from build123d import *

# Parameters (mm, degrees)
F0_R           = 0.875
F1_DEPTH       = 12.6
F2_DEPTH       = 2
F4_D           = 2
F4_DEPTH       = 38
F4_CBORE_D     = 3.5
F4_CBORE_DEPTH = 3
F4_TIP         = 0.600860619


# Not quite as in the source:
# - a feature names something its author has since deleted; it is built from what else it names


with BuildPart() as f1:
    # F0 (on Front) → F1 (new body)
    with BuildSketch(Plane.XZ):
        with BuildLine():
            Line((1, 0), (6.25, 0))
            Line((6.25, 0), (4.5, 17.15))
            Line((4.5, 17.15), (0, 17.15))
            Line((0, 17.15), (-4.5, 17.15))
            Line((-4.5, 17.15), (-6.25, 0))
            Line((-6.25, 0), (-1, 0))
            Line((-1, 0), (-1, 3))
            Line((-1, 3), (-3.25, 3))
            ThreePointArc((-3.25, 3), (-4.75, 4.5), (-3.25, 6))
            Line((-3.25, 6), (0, 6))
            Line((0, 6), (3.25, 6))
            ThreePointArc((3.25, 6), (4.75, 4.5), (3.25, 3))
            Line((3.25, 3), (1, 3))
            Line((1, 3), (1, 0))
        make_face()
        with Locations((-2.675, 9.625)):
            Circle(F0_R, mode=Mode.SUBTRACT)
        with Locations((2.675, 9.625)):
            Circle(F0_R, mode=Mode.SUBTRACT)
        with BuildLine():
            Line((-2.5, 16.4487531745), (0, 16.4487531745))
            Line((0, 16.4487531745), (2.5, 16.4487531745))
            ThreePointArc((2.5, 16.4487531745), (3.5, 15.4487531745), (2.5, 14.4487531745))
            Line((2.5, 14.4487531745), (0, 14.4487531745))
            Line((0, 14.4487531745), (-2.5, 14.4487531745))
            ThreePointArc((-2.5, 14.4487531745), (-3.5, 15.4487531745), (-2.5, 16.4487531745))
        make_face(mode=Mode.SUBTRACT)
        with BuildLine():
            Line((2.5, 16.4487531745), (0, 16.4487531745))
            Line((0, 16.4487531745), (-2.5, 16.4487531745))
            ThreePointArc((-2.5, 16.4487531745), (-3.5, 15.4487531745), (-2.5, 14.4487531745))
            Line((-2.5, 14.4487531745), (0, 14.4487531745))
            Line((0, 14.4487531745), (2.5, 14.4487531745))
            ThreePointArc((2.5, 14.4487531745), (3.5, 15.4487531745), (2.5, 16.4487531745))
        make_face()
        with Locations((-2.675, 9.625)):
            Circle(F0_R)
        with Locations((2.675, 9.625)):
            Circle(F0_R)
        with BuildLine():
            Line((1, 3.65), (1, 3))
            Line((1, 3), (3.25, 3))
            ThreePointArc((3.25, 3), (4.75, 4.5), (3.25, 6))
            Line((3.25, 6), (0, 6))
            Line((0, 6), (-3.25, 6))
            ThreePointArc((-3.25, 6), (-4.75, 4.5), (-3.25, 3))
            Line((-3.25, 3), (-1, 3))
            Line((-1, 3), (-1, 3.65))
            Line((-1, 3.65), (0, 3.65))
            Line((0, 3.65), (1, 3.65))
        make_face()
    extrude(amount=-F1_DEPTH)

    # F0 (on Front) → F2 (cut)
    with BuildSketch(Plane.XZ):
        with BuildLine():
            Line((1, 3.65), (1, 3))
            Line((1, 3), (3.25, 3))
            ThreePointArc((3.25, 3), (4.75, 4.5), (3.25, 6))
            Line((3.25, 6), (0, 6))
            Line((0, 6), (-3.25, 6))
            ThreePointArc((-3.25, 6), (-4.75, 4.5), (-3.25, 3))
            Line((-3.25, 3), (-1, 3))
            Line((-1, 3), (-1, 3.65))
            Line((-1, 3.65), (0, 3.65))
            Line((0, 3.65), (1, 3.65))
        make_face()
        with BuildLine():
            Line((2.5, 16.4487531745), (0, 16.4487531745))
            Line((0, 16.4487531745), (-2.5, 16.4487531745))
            ThreePointArc((-2.5, 16.4487531745), (-3.5, 15.4487531745), (-2.5, 14.4487531745))
            Line((-2.5, 14.4487531745), (0, 14.4487531745))
            Line((0, 14.4487531745), (2.5, 14.4487531745))
            ThreePointArc((2.5, 14.4487531745), (3.5, 15.4487531745), (2.5, 16.4487531745))
        make_face()
        with Locations((2.675, 9.625)):
            Circle(F0_R)
        with Locations((-2.675, 9.625)):
            Circle(F0_R)
    extrude(amount=-F2_DEPTH, mode=Mode.SUBTRACT)

    # F4
    with Locations(Plane.XY.offset(17.15)):
        with Locations((0, 6.3)):
            CounterBoreHole(F4_D / 2, F4_CBORE_D / 2, F4_CBORE_DEPTH, depth=F4_DEPTH)
            with Locations((0, 0, -(F4_DEPTH + F4_TIP / 2))):  # 118° drill point
                Cone(0, F4_D / 2, F4_TIP, mode=Mode.SUBTRACT)


solid = f1.part
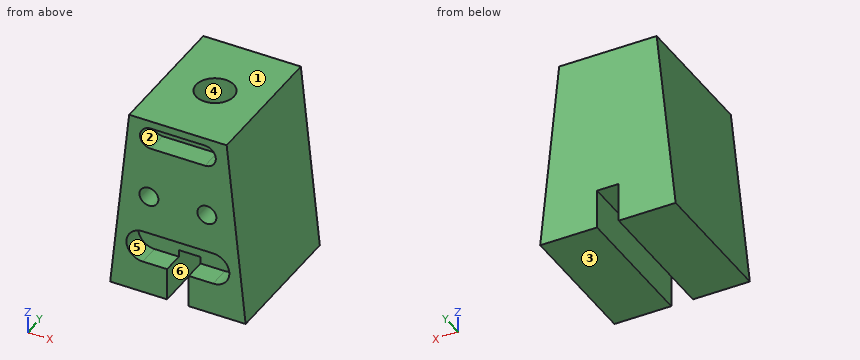
The model under review builds one solid part; all positions refer to its coordinate system, in mm. Face numbers are marked on the shaded views. A direction names the side the tool comes from. Give positions to 0.01 mm unless a question says otherwise; leave off trailing zeros. Write each loop counter-clockwise with the first axis right and the second up, starting at its lowest first coordinate (ties: lowest second). Pieces come first, ordered by that corner, then holes. Notation, with made-up numbers: M -35,84.25 L 18,84.25 A20 ccw 18,114.25 Z; hole C 78.5,60 d6. An arc over 180 degrees is marked long. One line per question, with ' | ' between items. Start each with the question number.
Item 1: For pin 1 (0.9 mm diameter, centred on x = -2.5, z = 9.5, fed in from -Y); pin 2 (6 mm diameter, centred on y = 1.5, z = 8.5, fed in from +X); pin 3 (4 mm diameter, centred on y = 8.5, z = 2.5, fed in from -X), all flat-tipped, find the tip position at first contact; note any pin that passes through.
Item 2: We need section A-A on x = 0. Write out the cut boundary in (y, z), plus the area to 3 significant figures.
Item 3: Draft analysis for pull direction Z (two halves, no side actions). For the marked faces 1, 2 and 3, state which applies: released by +Z, released by -Z, zero draft, split by the parting line, or undercut.
Item 4: We need section C-C on z = 5.5. Write out the cut boundary in (x, y), plus the area to 3 significant figures.
Item 5: We need section D-D on z = 2. Write out the cut boundary in (x, y), plus the area to 3 significant figures.
Item 6: For the marked faces 4, 5 and 6, list the 3-axis set-ups (+Z, -Z, +X, -X, +Y, -Y) from which the entire face can be reached by the end or side of a thin tool; tool diameter is ignored.
Item 7: We need section B-B on y = 10.75. Write out the cut boundary in (x, z).
Item 8: Wall thickness on line 1 (Y direction, x = 0, z = 12); line 2 (Z direction, x = 2.5, y = 1.75); line 3 (Y direction, x = 1.5, z = 3.5): over which ranges is each line inside the solid? List them lowest first. Write a range as from..to.
Results found:
1) pin 1: stops at y = 2 | pin 2: stops at x = 5.69 | pin 3: stops at x = -6.2
2) outline: M 0,6 L 2,6 L 2,3.65 L 5.3,3.65 L 5.3,14.15 L 4.55,14.15 L 4.55,17.15 L 0,17.15 L 0,16.45 L 2,16.45 L 2,14.45 L 0,14.45 Z; M 7.3,3.65 L 12.6,3.65 L 12.6,17.15 L 8.05,17.15 L 8.05,14.15 L 7.3,14.15 Z | area: 130 mm2
3) face 1: released by +Z | face 2: undercut | face 3: released by -Z
4) outline: M -5.69,0 L -4.37,0 L -4.37,2 L 4.37,2 L 4.37,0 L 5.69,0 L 5.69,12.6 L -5.69,12.6 Z; hole C 0,6.3 d2 | area: 123 mm2
5) outline: M -6.05,0 L -1,0 L -1,12.6 L -6.05,12.6 Z; M 1,0 L 6.05,0 L 6.05,12.6 L 1,12.6 Z | area: 127 mm2
6) face 4: +Z | face 5: -Y | face 6: -Z, +Y, -Y
7) outline: M -6.25,0 L -1,0 L -1,3.65 L 1,3.65 L 1,0 L 6.25,0 L 4.5,17.15 L -4.5,17.15 Z
8) line 1: y = 0..5.3, 7.3..12.6 | line 2: z = 0..3, 6..8.77, 10.48..14.45, 16.45..17.15 | line 3: y = 2..12.6
